The model under review builds one solid part; all positions refer to its coordinate system, in mm. Face numbers are marked on the shaded views. A direction names the side the tool comes from. Coordinates: 2 decimals unless noted, no trailing zeros. Write each loop counter-clockwise with the first axis right and the second up, starting at its lowest first coordinate (ties: lowest second). Pieces come first, ordered by that corner, then holes. Notation, with made-up numbers: M 58.25,44 L 100.25,44 A16 cw 100.25,53 Z; hole C -39,68.5 d8. An arc over 180 degrees is marked long. Answer as a JSON object with one key per item and string values.
Autodesk Inventor part; units mm, degrees
ref_plane "YZ Plane" through (0, 0, 0) normal (1, 0, 0) x (0, 1, 0)
ref_plane "XZ Plane" through (0, 0, 0) normal (0, 1, 0) x (-1, 0, 0)
ref_plane "XY Plane" through (0, 0, 0) normal (0, 0, 1) x (1, 0, 0)
sketch "Sketch1" plane through (0, 0, 0) normal (0, 1, 0) x (-1, 0, 0)
  line L0 (22, 14) -> (-22, 14)
  line L1 (-22, 14) -> (-22, 10)
  line L2 (-22, 10) -> (-2, 10)
  line L3 (-2, 10) -> (-2, -10)
  line L4 (-2, -10) -> (2, -10)
  line L5 (2, -10) -> (2, 10)
  line L6 (2, 10) -> (22, 10)
  line L7 (22, 10) -> (22, 14)
  point P0 (0, 0)
  point P1 (-2, 0)
  point P2 (0, 14)
  dimension "d0" = 20
  dimension "d1" = 4
  dimension "d2" = 20
  dimension "d3" = 4
  dimension "d4" = 20
extrude "Extrusion1" add sketch "Sketch1" along normal mid plane 15
sketch "Sketch2" plane through (-2, -7.5, 10) normal (0, 0, -1) x (-1, 0, 0)
  line L0 (20, 0) -> (0, 0)
  line L1 (20, 0) -> (20, 15)
  line L2 (0, 15) -> (20, 15)
  line L3 (0, 0) -> (0, 15)
  circle A0 centre (10, 7.5) radius 2.1
  point P0 (-2, 7.5)
  point P1 (20, 7.5)
  point P2 (10, 0)
  dimension "d7" = 4.2
extrude "Extrusion2" cut sketch "Sketch2" against normal up to next contours A0
sketch "Sketch3" plane through (2, -7.5, 10) normal (1, 0, 0) x (0, 0, -1)
  line L0 (20, 0) -> (0, 0)
  line L1 (20, 0) -> (20, 15)
  line L2 (0, 15) -> (20, 15)
  line L3 (0, 0) -> (0, 15)
  circle A0 centre (10, 7.5) radius 2.1
  point P0 (20, 7.5)
  point P1 (10, 0)
  dimension "d10" = 4.2
extrude "Extrusion3" cut sketch "Sketch3" against normal up to next contours A0
sketch "Sketch4" plane through (22, -7.5, 10) normal (0, 0, -1) x (-1, 0, 0)
  circle A0 centre (8, 7.5) radius 1.55
  line L0 (0, 0) -> (0, 15)
  point P0 (22, 7.5)
  point P1 (0, 7.5)
  dimension "d13" = 3.1
  dimension "d14" = 8
extrude "Extrusion4" cut sketch "Sketch4" against normal up to next
sketch "Sketch5" plane through (0, 7.5, 0) normal (0, 1, 0) x (1, 0, 0)
  line L0 (2, -4) -> (8, -10)
  line L1 (22, -10) -> (2, -10)
  line L2 (2, -10) -> (2, -4)
  line L3 (8, -10) -> (2, -10)
  point P0 (0, 0)
  dimension "d17" = 6
  dimension "d18" = 6
extrude "Extrusion5" add sketch "Sketch5" against normal blind 3
mirror "Mirror1" about plane through (0, 0, 0) normal (0, 1, 0) of "Extrusion5"
fillet "Fillet1" radius 2 4 edges at (-22, 7.5, 12) (22, 7.5, 12) (22, -7.5, 12) (-22, -7.5, 12)
sketch "Sketch6" plane through (8, 4.5, 10) normal (0, 0, -1) x (-1, 0, 0)
  point P0 (8, -4.5)
sketch "Sketch7" plane through (8, 4.5, 10) normal (0, 0, -1) x (-1, 0, 0)
  line L0 (-10.3107, -14.1904) -> (-16.6719, -14.1904)
  line L1 (-16.6719, -14.1904) -> (-16.6719, 4.7743)
  line L2 (-16.6719, 4.7743) -> (-10.3107, 4.7743)
  line L3 (-10.3107, 4.7743) -> (-10.3107, -14.1904)
  point P0 (8, -4.5)
extrude "Extrusion6" cut sketch "Sketch7" against normal up to next
fillet "Fillet2" radius 2 2 edges at (18.3107, 7.5, 12) (18.3107, -7.5, 12)
fillet "Fillet3" radius 2 6 edges at (0, -7.5, -10) (0, 7.5, -10) (2, 6, 4) (2, -6, 4) (8, 6, 10) (8, -6, 10)
properties part number "mount-heated-bed"
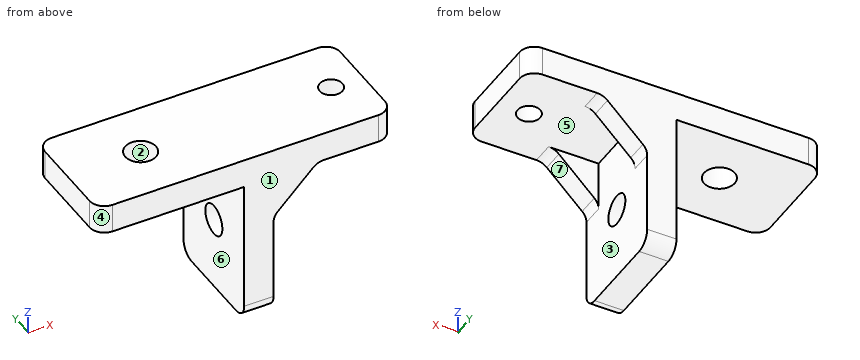
(1) Wall thickness on line 1 along Y through (x, z) = (-12, 12.6); line 2 along X through (y, z) = (-4, -3); line 3 along Z through (x, y) = (-8, -5): over which ranges is each line inside the solid? List them lowest first. Write a range as from..to.
Results list:
{"line 1": "-7.5..-2.1, 2.1..7.5", "line 2": "-2..2", "line 3": "10..14"}
(2) Add section A-A on y = 0. Give the boundary of the cut face in (x, z), and give its area (3 significant figures).
Results list:
{"outline": "M -22,10 L -14.1,10 L -14.1,14 L -22,14 Z; M -9.9,10 L -2,10 L -2,2.1 L 2,2.1 L 2,10 L 12.45,10 L 12.45,14 L -9.9,14 Z; M -2,-10 L 2,-10 L 2,-2.1 L -2,-2.1 Z; M 15.55,10 L 18.31,10 L 18.31,14 L 15.55,14 Z", "area": "195 mm²"}
(3) Add section C-C on x = 14. Give the boundary of the cut face in (y, z), and give its area (3 significant figures).
Results list:
{"outline": "M -7.5,10 L -1.55,10 L -1.55,14 L -7.5,14 Z; M 1.55,10 L 7.5,10 L 7.5,14 L 1.55,14 Z", "area": "47.6 mm²"}
(4) Add section D-D on z = 8.25. Give the boundary of the cut face in (x, y).
Results list:
{"outline": "M -2,-7.5 L 6.25,-7.5 L 6.25,-4.5 L 2,-4.5 L 2,4.5 L 6.25,4.5 L 6.25,7.5 L -2,7.5 Z"}
(5) For the marked faces 5, 6 and 7, list the 3-axis set-ups (+Z, -Z, +X, -X, +Y, -Y) from which the entire face can be reached by the end or side of a thin tool; tool diameter is ignored.
Results list:
{"face 5": "-Z, +X", "face 6": "-Z, -X, +Y, -Y", "face 7": "-Z, +X, +Y, -Y"}
(6) For pin 1 Ø1.5 at (y, z) = (-4, -0.5) entering from +X; pin 2 Ø6.5 at (x, y) = (-12, 0) entering from -Z; pin 3 Ø6.5 at (y, z) = (0, 0) entering from -X, all flat-tipped, find the tip position at first contact; note any pin that passes through.
Results list:
{"pin 1": "x = 2", "pin 2": "z = 10", "pin 3": "x = -2"}
(7) Add section B-B on z = 0. Give the boundary of the cut face in (x, y).
Results list:
{"outline": "M -2,-7.5 L 2,-7.5 L 2,-2.1 L -2,-2.1 Z; M -2,2.1 L 2,2.1 L 2,7.5 L -2,7.5 Z"}
(8) Draft analysis for pull direction X (two halves, no side actions). For the marked faces 1, 2, 3 and 4, state which applies: released by +X, released by -X, zero draft, split by the parting line, or undercut.
Results list:
{"face 1": "zero draft", "face 2": "undercut", "face 3": "released by +X", "face 4": "released by -X"}
